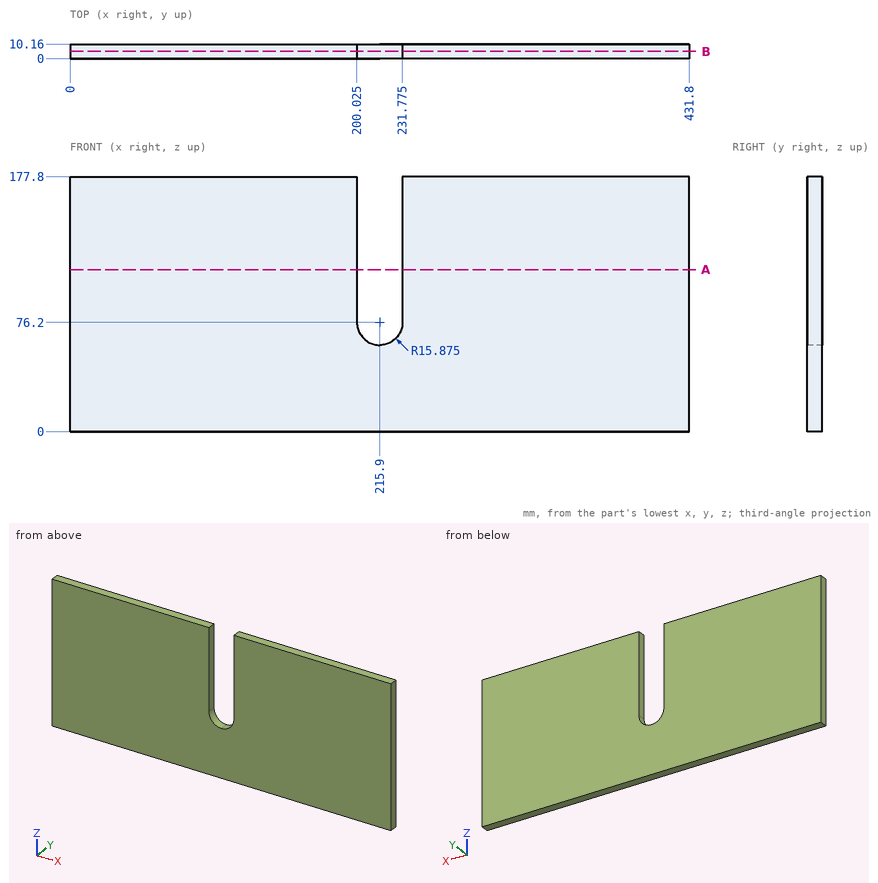
Source: three-view drawing plus pictorial views. Frame: mm from the lowest corner of the part. Coordinates: 2 decimals unless noted, no trailing zeros. Order: outer loops, then holes, each group sorted by start corner. A loop starts at its lowest first (then second) coordinate and runs counter-clockwise, first axis right, second up.
1) Section A-A (z = 113). Return loops of the section in (x, y) (3 decimals), then the cut area to 3 significant figures.
Result sheet:
outline: (0, 0) - (200.025, 0) - (200.025, 10.16) - (0, 10.16) - close; (231.775, 0) - (431.8, 0) - (431.8, 10.16) - (231.775, 10.16) - close
area: 4,060 mm2
2) First-contact query: P1, Ø8, axis at x = 143.5, z = 146.5, coming from the -Y side. Flat tip, straight axial feed; report the tip coordinate or a pass-through.
Result sheet:
P1: stops at y = 0
3) Section B-B (y = 5). Return loops of the section in (x, z) (3 decimals), then the cut area to 3 significant figures.
Result sheet:
outline: (0, 0) - (431.8, 0) - (431.8, 177.8) - (231.775, 177.8) - (231.775, 76.2) arc R15.875 cw to (215.9, 60.325) arc R15.875 cw to (200.025, 76.2) - (200.025, 177.8) - (0, 177.8) - close
area: 73,200 mm2
4) Ray query, probe 1 along X at (y, z) = (1.5, 126) (3 decimals); probe 2 along X at (y, z) = (5.5, 63); probe 3 along Z at (x, y) = (217, 3). Return the intervals inside material, ascending.
Result sheet:
probe 1: x = 0 to 200.025, 231.775 to 431.8
probe 2: x = 0 to 207.08, 224.72 to 431.8
probe 3: z = 0 to 60.36
